Build history of the part. All positions in model axes, mm. A direction names the side the tool comes from. Round coordinates to 2 decimals unless told otherwise and drop trailing zeros. Write each loop counter-clockwise with the first axis right and the second up, starting at its lowest first coordinate (ties: lowest second). Pieces come first, ordered by that corner, then holes. Notation, with made-up numbers: (88, -23.5) - (104, -23.5) arc R27 cw to (104, 1.5) - close; hole circle Ø6 at (26, 1.5). An arc over 180 degrees is marked (long way). One line per question, with ' | ' between items.
from build123d import *

# Parameters (mm, degrees)
ESQUISSE1_W             = 124
ESQUISSE1_H             = 66
ESQUISSE1_W_2           = 119
ESQUISSE1_H_2           = 61
BOSS_EXTRU_1_DEPTH      = 15
ESQUISSE2_W             = 124
ESQUISSE2_H             = 30
BOSS_EXTRU_2_DEPTH      = 5
ESQUISSE3_W             = 124
ESQUISSE3_H             = 30
BOSS_EXTRU_3_DEPTH      = 5
ESQUISSE2_4_W           = 119
ESQUISSE2_4_H           = 33.5
ENL_V_MAT_EXTRU_2_DEPTH = 139.544216769
ESQUISSE4_W             = 124
ESQUISSE4_H             = 5
BOSS_EXTRU_4_DEPTH      = 10
ESQUISSE6_W             = 124
ESQUISSE6_H             = 5
BOSS_EXTRU_5_DEPTH      = 10
ESQUISSE5_W             = 40
ESQUISSE5_H             = 2.5
ENL_V_MAT_EXTRU_3_DEPTH = 10
CONG_5_R                = 5
CONG_6_R                = 3.5
CONG_7_R                = 1.25
ESQUISSE7_W             = 37
ESQUISSE7_H             = 15
ENL_V_MAT_EXTRU_4_DEPTH = 129.134694755


with BuildPart() as part:
    # Esquisse1 → Boss.-Extru.1 (new body)
    with BuildSketch(Plane.XY):
        with Locations((59.5, 30.5)):
            Rectangle(ESQUISSE1_W, ESQUISSE1_H)
        with Locations((59.5, 30.5)):
            Rectangle(ESQUISSE1_W_2, ESQUISSE1_H_2, mode=Mode.SUBTRACT)
    extrude(amount=BOSS_EXTRU_1_DEPTH)

    # Esquisse2 → Boss.-Extru.2 (add)
    with BuildSketch(Plane.XY.offset(15)):
        with Locations((59.5, 12.5)):
            Rectangle(ESQUISSE2_W, ESQUISSE2_H)
    extrude(amount=BOSS_EXTRU_2_DEPTH)

    # Esquisse3 → Boss.-Extru.3 (add)
    with BuildSketch(Plane(origin=(0, 0, 0), x_dir=(-1, 0, 0), z_dir=(0, 0, -1))):
        with Locations((-59.5, 12.5)):
            Rectangle(ESQUISSE3_W, ESQUISSE3_H)
    extrude(amount=BOSS_EXTRU_3_DEPTH)

    # Esquisse2<4> → Enlèv. mat.-Extru.2 (cut, through all)
    with BuildSketch(Plane.XY.offset(15)):
        Polygon((-2.5, 63.5), (-2.5, 27.5), (0, 27.5), (0, 61), (119, 61), (119, 27.5), (121.5, 27.5), (121.5, 63.5), align=None)
        with Locations((59.5, 44.25)):
            Rectangle(ESQUISSE2_4_W, ESQUISSE2_4_H)
        Polygon((-7.324686497, 27.5), (-2.5, 27.5), (-2.5, 63.5), (121.5, 63.5), (121.5, 27.5), (134.265191069, 27.5), (134.265191069, 70.183408252), (-7.324686497, 70.183408252), align=None)
    extrude(amount=-ENL_V_MAT_EXTRU_2_DEPTH, mode=Mode.SUBTRACT)

    # Esquisse4 → Boss.-Extru.4 (add)
    with BuildSketch(Plane.XY.offset(20)):
        with Locations((59.5, 25)):
            Rectangle(ESQUISSE4_W, ESQUISSE4_H)
    extrude(amount=BOSS_EXTRU_4_DEPTH)

    # Esquisse6 → Boss.-Extru.5 (add)
    with BuildSketch(Plane(origin=(0, 0, -5), x_dir=(-1, 0, 0), z_dir=(0, 0, -1))):
        with Locations((-59.5, 25)):
            Rectangle(ESQUISSE6_W, ESQUISSE6_H)
    extrude(amount=BOSS_EXTRU_5_DEPTH)

    # Esquisse5 → Enlèv. mat.-Extru.3 (cut)
    with BuildSketch(Plane(origin=(0, 27.5, 0), x_dir=(1, 0, 0), z_dir=(0, 1, 0))):
        with Locations((22.5, -25.25)):
            Rectangle(ESQUISSE5_W, ESQUISSE5_H)
        with Locations((96.5, -25.25)):
            Rectangle(ESQUISSE5_W, ESQUISSE5_H)
        with Locations((22.5, 10.25)):
            Rectangle(ESQUISSE5_W, ESQUISSE5_H)
        with Locations((96.5, 10.25)):
            Rectangle(ESQUISSE5_W, ESQUISSE5_H)
    extrude(amount=-ENL_V_MAT_EXTRU_3_DEPTH, mode=Mode.SUBTRACT)

    # Congé5
    cong_5_edges = [part.edges().sort_by_distance(p)[0] for p in [
        (121.5, 25, 30),
        (121.5, 25, -15),
        (-2.5, 25, -15),
        (-2.5, 25, 30),
    ]]
    fillet(cong_5_edges, radius=CONG_5_R)

    # Congé6
    cong_6_edges = [part.edges().sort_by_distance(p)[0] for p in [
        (59.5, 22.5, 20),
        (59.5, 22.5, -5),
    ]]
    fillet(cong_6_edges, radius=CONG_6_R)

    # Congé7
    cong_7_edges = [part.edges().sort_by_distance(p)[0] for p in [
        (76.5, 25, -11.5),
        (76.5, 25, -9),
        (116.5, 25, -9),
        (116.5, 25, -11.5),
        (42.5, 25, -11.5),
        (42.5, 25, -9),
        (2.5, 25, -11.5),
        (2.5, 25, -9),
        (2.5, 25, 24),
        (2.5, 25, 26.5),
        (42.5, 25, 24),
        (42.5, 25, 26.5),
        (76.5, 25, 24),
        (76.5, 25, 26.5),
        (116.5, 25, 24),
        (116.5, 25, 26.5),
    ]]
    fillet(cong_7_edges, radius=CONG_7_R - 0.0001)  # a hair under: the kernel refuses the full size

    # Esquisse7 → Enlèv. mat.-Extru.4 (cut, through all)
    with BuildSketch(Plane(origin=(0, 0, 0), x_dir=(1, 0, 0), z_dir=(0, 1, 0))):
        with Locations((97.5, -7.5)):
            Rectangle(ESQUISSE7_W, ESQUISSE7_H)
    extrude(amount=-ENL_V_MAT_EXTRU_4_DEPTH, mode=Mode.SUBTRACT)


solid = part.part
Q1. Saw through at C-C, the plane y = 20.5. List the corners of the cut face in (x, z).
Found:
outline: (-2.5, -5.34) - (121.5, -5.34) - (121.5, 20.34) - (-2.5, 20.34) - close; hole (0, 0) - (119, 0) - (119, 15) - (0, 15) - close
Q2. Drop flat-ended pins along their axis: pin 1 (11 mm diameter, centred on x = 49, y = 5, fed in from -Z); pin 2 (12 mm diameter, centred on x = 94, y = 3, fed in from +Z); pin 3 (6 mm diameter, centred on x = 72.5, z = 21, fed in from -Y); pin 4 (5 mm diameter, centred on y = 14, z = -8, fed in from -X). Give the stop position or say it passes through.
Found:
pin 1: z = -5 | pin 2: z = 20 | pin 3: y = -2.5 | pin 4: through
Q3. Saw through at B-B, the plane x = 88.5. List the corners of the cut face in (y, z).
Found:
outline: (-2.5, -5) - (19, -5) arc R3.5 cw to (22.5, -8.5) - (22.5, -9) - (27.5, -9) - (27.5, 0) - (-2.5, 0) - close; (-2.5, 15) - (27.5, 15) - (27.5, 24) - (22.5, 24) - (22.5, 23.5) arc R3.5 cw to (19, 20) - (-2.5, 20) - close; (22.5, -15) - (27.5, -15) - (27.5, -11.5) - (22.5, -11.5) - close; (22.5, 26.5) - (27.5, 26.5) - (27.5, 30) - (22.5, 30) - close
Q4. Pull direction Z, two halves, no side cores. Call faces 1 (the cylindrical face through (-1, 25.04, -13.57)), 2 (the flat face through (22, 25, 24)), 3 (the flat face through (-2.5, 12, 8)): +Z half, -Z half, draft (parallel to the pull), parting line (faces both ways), or undercut.
Found:
face 1: -Z half | face 2: undercut | face 3: draft
Q5. Saw through at A-A, the plane z = 5. List the corners of the cut face in (x, y).
Found:
outline: (-2.5, -2.5) - (79, -2.5) - (79, 0) - (0, 0) - (0, 27.5) - (-2.5, 27.5) - close; (116, -2.5) - (121.5, -2.5) - (121.5, 27.5) - (119, 27.5) - (119, 0) - (116, 0) - close
Q6. Drill centre lines: L1, parallel to Z at x = 32, y = 25; L2, parallel to Z at x = 22, y = 11.5; L3, parallel to X at y = 16.25, z = 7. Where is each one in solid material? Low to high. Write a range as from..to.
Found:
L1: -15..-11.5, -9..0, 15..24, 26.5..30 | L2: -5..0, 15..20 | L3: -2.5..0, 119..121.5
Q7. Which spindle directions (+Z, -Z, +X, -X, +Y, -Y) get a long thin tool onto all of the face, cutting with end or side? Do faces 4 (the flat face through (60, 22.5, -12)), 5 (the flat face through (116, -1, 8)), 6 (the flat face through (0, 14, 7)), 7 (the flat face through (59, 8, 20)). Say none if no direction does.
Found:
face 4: -Z, +X, -X, -Y | face 5: +Y, -Y | face 6: +Y | face 7: +Z, +X, -X, -Y
Q8. Saw through at D-D, the plane x = 12.5. List the corners of the cut face in (y, z).
Found:
outline: (-2.5, -5) - (19, -5) arc R3.5 cw to (22.5, -8.5) - (22.5, -9) - (27.5, -9) - (27.5, 0) - (0, 0) - (0, 15) - (27.5, 15) - (27.5, 24) - (22.5, 24) - (22.5, 23.5) arc R3.5 cw to (19, 20) - (-2.5, 20) - close; (22.5, -15) - (27.5, -15) - (27.5, -11.5) - (22.5, -11.5) - close; (22.5, 26.5) - (27.5, 26.5) - (27.5, 30) - (22.5, 30) - close
